```python
from build123d import *

# Parameters (mm, degrees)
F1_DEPTH  = 50.8
F3_DEPTH  = 12.701
F5_DEPTH  = 12.7
F6_DEPTH  = 12.701
F7_R      = 6.35
F8_DEPTH  = 25.401
F9_R      = 3.175
F10_DEPTH = 6.351
F12_DEPTH = 6.351


with BuildPart() as f1:
    # F0 (on Right) → F1 (new body)
    with BuildSketch(Plane.YZ):
        Polygon((12.7, 0), (12.7, 63.5), (0, 63.5), (0, 6.35), (-19.05, 6.35), (-19.05, 0), align=None)
    extrude(amount=F1_DEPTH)

    # F2 (on face) → F3 (cut, through all)
    with BuildSketch(Plane.XZ):
        with BuildLine():
            Line((12.7, 19.05), (12.7, 63.5))
            Line((12.7, 63.5), (0, 63.5))
            Line((0, 63.5), (0, 31.75))
            ThreePointArc((0, 31.75), (8.9802561211, 28.0302561211), (12.7, 19.05))
        make_face()
        with BuildLine():
            Line((38.1, 63.5), (38.1, 19.05))
            ThreePointArc((38.1, 19.05), (41.8197438789, 28.0302561211), (50.8, 31.75))
            Line((50.8, 31.75), (50.8, 63.5))
            Line((50.8, 63.5), (38.1, 63.5))
        make_face()
        with BuildLine():
            Line((0, 31.75), (0, 6.35))
            ThreePointArc((0, 6.35), (8.9802561211, 10.0697438789), (12.7, 19.05))
            ThreePointArc((12.7, 19.05), (8.9802561211, 28.0302561211), (0, 31.75))
        make_face()
        with BuildLine():
            ThreePointArc((50.8, 31.75), (41.8197438789, 28.0302561211), (38.1, 19.05))
            ThreePointArc((38.1, 19.05), (41.8197438789, 10.0697438789), (50.8, 6.35))
            Line((50.8, 6.35), (50.8, 31.75))
        make_face()
    extrude(amount=-F3_DEPTH, mode=Mode.SUBTRACT)

    # F4 (on face) → F5 (join)
    with BuildSketch(Plane.XZ):
        with BuildLine():
            ThreePointArc((12.7, 50.8), (25.4, 38.1), (38.1, 50.8))
            ThreePointArc((38.1, 50.8), (34.3802561211, 59.7802561211), (25.4, 63.5))
            ThreePointArc((25.4, 63.5), (16.4197438789, 59.7802561211), (12.7, 50.8))
        make_face()
    extrude(amount=F5_DEPTH)

    # F6 (cut, through all): faces of the model
    f6_faces = [f1.faces().sort_by_distance(p)[0] for p in [
        (15.5367728246, 0, 60.6632271754),
        (35.2632271754, 0, 60.6632271754),
    ]]
    extrude(f6_faces, amount=-F6_DEPTH, mode=Mode.SUBTRACT)

    # F7 (on face) → F8 (cut, through all)
    with BuildSketch(Plane.XZ.offset(12.7)):
        with Locations((25.4, 50.8)):
            Circle(F7_R)
    extrude(amount=-F8_DEPTH, mode=Mode.SUBTRACT)

    # F9 (on face) → F10 (cut, through all)
    with BuildSketch(Plane.XY.offset(6.35)):
        with Locations((9.525, -9.525)):
            Circle(F9_R)
        with Locations((41.275, -9.525)):
            Circle(F9_R)
    extrude(amount=-F10_DEPTH, mode=Mode.SUBTRACT)

    # F11 (on face) → F12 (cut, through all)
    with BuildSketch(Plane.XY.offset(6.35)):
        with BuildLine():
            Line((0, -19.05), (12.7, -19.05))
            ThreePointArc((12.7, -19.05), (3.7197438789, -15.3302561211), (0, -6.35))
            Line((0, -6.35), (0, -19.05))
        make_face()
        with BuildLine():
            ThreePointArc((50.8, -6.35), (47.0802561211, -15.3302561211), (38.1, -19.05))
            Line((38.1, -19.05), (50.8, -19.05))
            Line((50.8, -19.05), (50.8, -6.35))
        make_face()
    extrude(amount=-F12_DEPTH, mode=Mode.SUBTRACT)


solid = f1.part
```
Part model, mm, in its own coordinate system. A direction names the side the tool comes from. Give positions to 0.01 mm unless a question says otherwise; leave off trailing zeros. Write each loop counter-clockwise with the first axis right and the second up, starting at its lowest first coordinate (ties: lowest second). Pieces come first, ordered by that corner, then holes. Notation, with made-up numbers: (-11, -12) -> (37, -12) arc R20 cw to (37, -8) -> close; hole circle Ø2 at (79, 44.25). An arc over 180 degrees is marked (long way). Put each result on its own line as item: value. Start each with the question number.
Item 1: Cut at A-A (y = -5). List the corners of the cut face in (x, z), then the cut area to 3 significant figures.
Item 2: Cut at B-B (x = 30.5). List the corners of the cut face in (y, z).
Item 3: Cut at C-C (y = 1). List the corners of the cut face in (x, z).
Item 4: Pin check, flat tips, straight feed: pin 1 Ø8 at (x, y) = (14.5, 1.5) entering from +Z; pin 2 Ø10 at (y, z) = (4.5, 40.5) entering from -X; pin 3 Ø7.5 at (x, z) = (21.5, 56) entering from -Y. Stop position of each tip, or through.
Item 5: Cut at D-D (z = 5.5). List the corners of the cut face in (x, y) (3 decimals), then the cut area to 3 significant figures.
Item 6: Which spindle directions (+Z, -Z, +X, -X, +Y, -Y) get a long thin tool onto all of the face, cutting with end or side? Do faces 1 (the face through (38.1, 6, 35)), 2 (the face through (28, -12.7, 57)), 3 (the face through (12.7, 6, 35)). Say none if no direction does.
Item 7: Wall check: L1, parallel to X at y = 6, z = 23; L2, parallel to Z at x = 6, y = -14; L3, parallel to Z at x = 25.4, y = 1. Give the ranges that are in metal, low to high. Write a range as [from, to].
Item 8: Pull direction Z, two halves, no side cores. Call faces 4 (the face through (25, -3, 0)), 5 (the face through (12.46, -10.74, 3.22)), 6 (the face through (24.6, -0.2, 57.1)): pulls with the +Z half, pulls with the -Z half, needs draft (parallel to the pull), parting line crosses it, or undercut.
Answer list:
1. outline: (0, 0) -> (50.8, 0) -> (50.8, 6.35) -> (0, 6.35) -> close; circle Ø25.4 at (25.4, 50.8); hole circle Ø12.7 at (25.4, 50.8)
1. area: 703 mm2
2. outline: (-19.05, 0) -> (12.7, 0) -> (12.7, 47.02) -> (-12.7, 47.02) -> (-12.7, 39.17) -> (0, 39.17) -> (0, 6.35) -> (-19.05, 6.35) -> close; (-12.7, 54.58) -> (12.7, 54.58) -> (12.7, 62.43) -> (-12.7, 62.43) -> close
3. outline: (0, 0) -> (50.8, 0) -> (50.8, 6.35) arc R12.7 cw to (38.1, 19.05) -> (38.1, 50.8) arc R12.7 ccw to (12.7, 50.8) -> (12.7, 19.05) arc R12.7 cw to (0, 6.35) -> close; hole circle Ø12.7 at (25.4, 50.8)
4. pin 1: stops at z = 61.46
4. pin 2: stops at x = 12.7
4. pin 3: stops at y = -12.7
5. outline: (0, -6.35) arc R12.7 ccw to (12.7, -19.05) -> (38.1, -19.05) arc R12.7 ccw to (50.8, -6.35) -> (50.8, 12.7) -> (0, 12.7) -> close; hole circle Ø6.35 at (9.525, -9.525); hole circle Ø6.35 at (41.275, -9.525)
5. area: 1,480 mm2
6. face 1: +Z, +X, +Y, -Y
6. face 2: +Z, +X, -X, -Y
6. face 3: +Z, -X, +Y, -Y
7. L1: x = [12.7, 38.1]
7. L2: z = [0, 6.35]
7. L3: z = [0, 44.45], [57.15, 63.5]
8. face 4: pulls with the -Z half
8. face 5: needs draft
8. face 6: undercut
